Design review of the part built by this model. Coordinates are the model's own, in mm. A direction names the side the tool comes from. Round coordinates to 2 decimals unless told otherwise and drop trailing zeros. Loops run counter-clockwise (first coordinate to the right, second up) from the corner with the lowest first, then second, coordinate; pieces in that order, holes last. Notation, with made-up numbers: (-26.5, 30.5) -> (-4.5, 30.5) arc R32 ccw to (-4.5, 56.5) -> close; hole circle Ø5 at (-13, 68). An arc over 180 degrees is marked (long way). Answer as CSV lines item,"result". Start each with the question number.
(1) Take a section at C-C, the plane z = 0. Write out the cut boundary in (x, y), and give its area (3 significant figures).
(2) Machinability: for faces 1 (the face through (0, 0, 0)), 2 (the face through (0, 4, 6.5)), 3 (the face through (10.7, 4, -3)), which of the approach directions +Z, -Z, +X, -X, +Y, -Y give a long, thin tool a straight path to every point of the face, cutting with its end or side? Answer none if there is none.
(3) Draft analysis for pull direction Z (two halves, no side actions). For faces 4 (the face through (0, 3, 7.3)), 5 (the face through (11.5, 2, -2)), 6 (the face through (11, 4, 0.5)), 7 (the face through (0, 3, -7.3)), state which applies: +Z half, -Z half, draft (parallel to the pull), parting line (faces both ways), or undercut.
(4) To check wall thickness, follow line 1 (X direction, y = 0.9, z = 0); line 2 (Z direction, x = -5.5, y = 3.35); line 3 (Y direction, x = -4.25, z = -3.5). State the ranges of each line that lie inside material, in increasing order. Write a range as from..to.
(5) Take a section at B-B, the plane y = 3.7. Write out the cut boundary in (x, z), and give its area (3 significant figures).
(6) For P1, Ø0.7, axis at y = 4, z = -2.5, coming from the -X side; P2, Ø1.5, axis at x = 8.5, z = 3.5, coming from the +Y side, all flat-tipped, find the tip position at first contact; note any pin that passes through.
(7) Take a section at D-D, the plane x = 8.5. Write out the cut boundary in (y, z), and give its area (3 significant figures).
(8) Take a section at A-A, the plane x = -7.3. Write out the cut boundary in (y, z), and give its area (3 significant figures).
from build123d import *

# Parameters (mm, degrees)
SKETCH1_W           = 23
SKETCH1_H           = 14.6
BOSS_EXTRUDE1_DEPTH = 3
SKETCH2_R           = 1.2
CUT_EXTRUDE1_DEPTH  = 14.947759677
SKETCH3_W           = 23
SKETCH3_H           = 0.8
BOSS_EXTRUDE2_DEPTH = 2.4


with BuildPart() as part:
    # Sketch1 → Boss-Extrude1 (new body)
    with BuildSketch(Plane(origin=(0, 0, 0), x_dir=(1, 0, 0), z_dir=(0, 1, 0))):
        Rectangle(SKETCH1_W, SKETCH1_H)
    extrude(amount=BOSS_EXTRUDE1_DEPTH)

    # Sketch2 → Cut-Extrude1 (cut, through all)
    with BuildSketch(Plane(origin=(0, 3, 0), x_dir=(1, 0, 0), z_dir=(0, 1, 0))):
        with Locations(Location((-7.3, 0, 0), (0, 0, 270))):
            Circle(SKETCH2_R)
    extrude(amount=-CUT_EXTRUDE1_DEPTH, mode=Mode.SUBTRACT)

    # Sketch3 → Boss-Extrude2 (add)
    with BuildSketch(Plane(origin=(0, 3, 0), x_dir=(1, 0, 0), z_dir=(0, 1, 0))):
        Polygon((-11.5, 7.3), (11.5, 7.3), (11.5, -0.5), (10.7, -0.5), (10.7, 6.5), (-11.5, 6.5), align=None)
        with Locations((0, -6.9)):
            Rectangle(SKETCH3_W, SKETCH3_H)
    extrude(amount=BOSS_EXTRUDE2_DEPTH)


solid = part.part
The answers:
1,outline,"(-11.5, 0) -> (-8.5, 0) -> (-8.5, 3) -> (-11.5, 3) -> close; (-6.1, 0) -> (11.5, 0) -> (11.5, 5.4) -> (10.7, 5.4) -> (10.7, 3) -> (-6.1, 3) -> close"
1,area,"63.7 mm²"
2,face 1,"+Z, -Z, +X, -X, -Y"
2,face 2,"+X, -X, +Y"
2,face 3,"-X, +Y"
3,face 4,"+Z half"
3,face 5,"draft"
3,face 6,"undercut"
3,face 7,"-Z half"
4,line 1,"-11.5..-8.5, -6.1..11.5"
4,line 2,"-7.3..-6.5, 6.5..7.3"
4,line 3,"0..3"
5,outline,"(-11.5, -7.3) -> (11.5, -7.3) -> (11.5, 0.5) -> (10.7, 0.5) -> (10.7, -6.5) -> (-11.5, -6.5) -> close; (-11.5, 6.5) -> (11.5, 6.5) -> (11.5, 7.3) -> (-11.5, 7.3) -> close"
5,area,"42.4 mm²"
6,P1,"x = 10.7"
6,P2,"y = 3"
7,outline,"(0, -7.3) -> (5.4, -7.3) -> (5.4, -6.5) -> (3, -6.5) -> (3, 6.5) -> (5.4, 6.5) -> (5.4, 7.3) -> (0, 7.3) -> close"
7,area,"47.6 mm²"
8,outline,"(0, -7.3) -> (5.4, -7.3) -> (5.4, -6.5) -> (3, -6.5) -> (3, -1.2) -> (0, -1.2) -> close; (0, 1.2) -> (3, 1.2) -> (3, 6.5) -> (5.4, 6.5) -> (5.4, 7.3) -> (0, 7.3) -> close"
8,area,"40.4 mm²"
